For this review, take the finished solid that the model builds, in its own axes (mm). Face numbers are marked on the shaded views. A direction names the side the tool comes from. Coordinates: 2 decimals unless noted, no trailing zeros. Write each loop counter-clockwise with the first axis right and the second up, starting at its lowest first coordinate (ties: lowest second). Pieces come first, ordered by that corner, then holes.
1) We need section B-B on z = 32. Write out the cut boundary in (x, y), then the cut area to 3 significant figures.
2) We need section A-A on y = 0. Write out the cut boundary in (x, z), then the cut area to 3 significant figures.
3) We need section C-C on x = 73.5. Write out the cut boundary in (y, z).
4) We need section D-D on y = 67. Write out the cut boundary in (x, z).
5) Insertion check: P1, Ø8, axis at y = 56.5, z = 36.5, coming from the +X side; P2, Ø23.5, axis at x = 0, y = 0, coming from the -Z side; P3, Ø3, axis at x = -13, z = 6, coming from the -Y side; P4, Ø6, axis at x = -8.5, z = 33.5, coming from the -Y side. Each pin has a flat end and moves straight along its axis. Give the tip position at first contact, or say it passes through.
6) Mouldability with a two-part tool opening along Z and no side actions: class the marked faces 1, 2, 3 and 4 as pulls with the +Z half, pulls with the -Z half, needs draft (parallel to the pull), parting line crosses it, or undercut.
7) For the marked faces 5, 6, 7, 8 and 9, list the 3-axis set-ups (+Z, -Z, +X, -X, +Y, -Y) from which the entire face can be reached by the end or side of a thin tool; tool diameter is ignored.
8) To check wall thickness, follow line 1 along X through (y, z) = (-8, 46); line 2 along Y through (x, z) = (54, 7.5); line 3 along Z through (x, y) = (3, -2.5). State the ranges of each line that lie inside material, in increasing order.
from build123d import *

# Parameters (mm, degrees)
SKIZZE1_W                       = 50
SKIZZE1_H                       = 50
SKIZZE1_R                       = 45
AUFSATZ_LINEAR_AUSTRAGEN2_DEPTH = 55
SCHNITT_LINEAR_AUSTRAGEN1_DEPTH = 43
SKIZZE4_R                       = 1.5
SCHNITT_LINEAR_AUSTRAGEN2_DEPTH = 10
SKIZZE5_R                       = 3.5
SCHNITT_LINEAR_AUSTRAGEN3_DEPTH = 4.5
SCHNITT_LINEAR_AUSTRAGEN4_DEPTH = 21
SCHNITT_LINEAR_START            = -6
SKIZZE7_R                       = 13
SCHNITT_LINEAR_AUSTRAGEN5_DEPTH = 49
SKIZZE8_R                       = 12
SCHNITT_LINEAR_AUSTRAGEN6_DEPTH = 165.772570533
SKIZZE9_R                       = 1.65
SCHNITT_LINEAR_AUSTRAGEN9_DEPTH = 20


with BuildPart() as part:
    # Skizze1 → Aufsatz-Linear austragen2 (new body)
    with BuildSketch(Plane.XY):
        with BuildLine():
            Line((35, 35), (35, 85))
            Line((35, 85), (-27.896103401, 35.310160224))
            ThreePointArc((-27.896103401, 35.310160224), (19.617279971, 40.498917597), (45, 0))
            ThreePointArc((45, 0), (31.819805153, -31.819805153), (0, -45))
            Line((0, -45), (85, -45))
            Line((85, -45), (85, 35))
            Line((85, 35), (35, 35))
        make_face()
        with Locations((60, 60)):
            Rectangle(SKIZZE1_W, SKIZZE1_H)
        Circle(SKIZZE1_R)
    extrude(amount=AUFSATZ_LINEAR_AUSTRAGEN2_DEPTH)

    # Skizze3 → Schnitt-Linear austragen1 (cut)
    with BuildSketch(Plane.XZ.offset(45)):
        Polygon((60, 48.5), (19, 48.5), (19, 6.5), (60, 6.5), (60, 16.5), (70, 16.5), (70, 6.5), (85, 6.5), (85, 48.5), (70, 48.5), (70, 38.5), (60, 38.5), align=None)
    extrude(amount=-SCHNITT_LINEAR_AUSTRAGEN1_DEPTH, mode=Mode.SUBTRACT)

    # Skizze4 → Schnitt-Linear austragen2 (cut)
    with BuildSketch(Plane(origin=(70, 0, 0), x_dir=(0, 0, -1), z_dir=(1, 0, 0))):
        with Locations(Location((-42.999780644, -7.500219356, 0), (0, 0, 90))):
            Circle(SKIZZE4_R)
        with Locations(Location((-12.000219356, -7.500219356, 0), (0, 0, 90))):
            Circle(SKIZZE4_R)
        with Locations(Location((-12.000219356, -38.499780644, 0), (0, 0, 90))):
            Circle(SKIZZE4_R)
        with BuildLine():
            ThreePointArc((-41.499780644, -38.499780644), (-42.402127924, -37.123985882), (-44.023528946, -37.403450669))
            ThreePointArc((-44.023528946, -37.403450669), (-42.999780644, -38.499780644), (-41.903450669, -39.523528946))
            ThreePointArc((-41.903450669, -39.523528946), (-41.604342547, -39.050010158), (-41.499780644, -38.499780644))
        make_face()
        with BuildLine():
            ThreePointArc((-41.903450669, -39.523528946), (-42.999780644, -38.499780644), (-44.023528946, -37.403450669))
            ThreePointArc((-44.023528946, -37.403450669), (-44.060440815, -39.560440815), (-41.903450669, -39.523528946))
        make_face()
    extrude(amount=-SCHNITT_LINEAR_AUSTRAGEN2_DEPTH, mode=Mode.SUBTRACT)

    # Skizze5 → Schnitt-Linear austragen3 (cut)
    with BuildSketch(Plane(origin=(70, 0, 0), x_dir=(0, 0, -1), z_dir=(1, 0, 0))):
        with Locations(Location((-42.999780644, -7.500219356, 0), (0, 0, 90))):
            Circle(SKIZZE5_R)
        with Locations(Location((-12.000219356, -7.500219356, 0), (0, 0, 90))):
            Circle(SKIZZE5_R)
        with Locations(Location((-12.000219356, -38.499780644, 0), (0, 0, 90))):
            Circle(SKIZZE5_R)
        with Locations(Location((-42.999780644, -38.499780644, 0), (0, 0, 90))):
            Circle(SKIZZE5_R)
    extrude(amount=-SCHNITT_LINEAR_AUSTRAGEN3_DEPTH, mode=Mode.SUBTRACT)

    # Skizze6 → Schnitt-Linear austragen4 (cut, symmetric)
    with BuildSketch(Plane.XY.offset(27.5)):
        Polygon((29, 10.5), (19, 10.5), (19, 3), (19, -2), (29, -2), align=None)
        with BuildLine():
            Line((19, 3), (19, 10.5))
            Line((19, 10.5), (5.809475019, 10.5))
            ThreePointArc((5.809475019, 10.5), (9.486832981, 7.348469228), (11.618950039, 3))
            Line((11.618950039, 3), (19, 3))
        make_face()
    extrude(amount=SCHNITT_LINEAR_AUSTRAGEN4_DEPTH, both=True, mode=Mode.SUBTRACT)

    # Skizze7 → Schnitt-Linear austragen5 (cut)
    with BuildSketch(Plane.XY.offset(55).offset(SCHNITT_LINEAR_START)):
        Circle(SKIZZE7_R)
    extrude(amount=-SCHNITT_LINEAR_AUSTRAGEN5_DEPTH, mode=Mode.SUBTRACT)

    # Skizze8 → Schnitt-Linear austragen6 (cut, through all)
    with BuildSketch(Plane(origin=(85, 0, 0), x_dir=(0, 0, -1), z_dir=(1, 0, 0))):
        with Locations(Location((-27.5, 57.5, 0), (0, 0, 90))):
            Circle(SKIZZE8_R)
    extrude(amount=-SCHNITT_LINEAR_AUSTRAGEN6_DEPTH, mode=Mode.SUBTRACT)

    # Skizze9 → Schnitt-Linear austragen9 (cut)
    with BuildSketch(Plane(origin=(0, 0, 0), x_dir=(-1, 0, 0), z_dir=(0, 0, -1))):
        with Locations((-10.037587636, 14.335160775)):
            Circle(SKIZZE9_R)
        with Locations((14.335160775, 10.037587636)):
            Circle(SKIZZE9_R)
        with Locations((10.037587636, -14.335160775)):
            Circle(SKIZZE9_R)
        with Locations((-14.335160775, -10.037587636)):
            Circle(SKIZZE9_R)
    extrude(amount=-SCHNITT_LINEAR_AUSTRAGEN9_DEPTH, mode=Mode.SUBTRACT)


solid = part.part
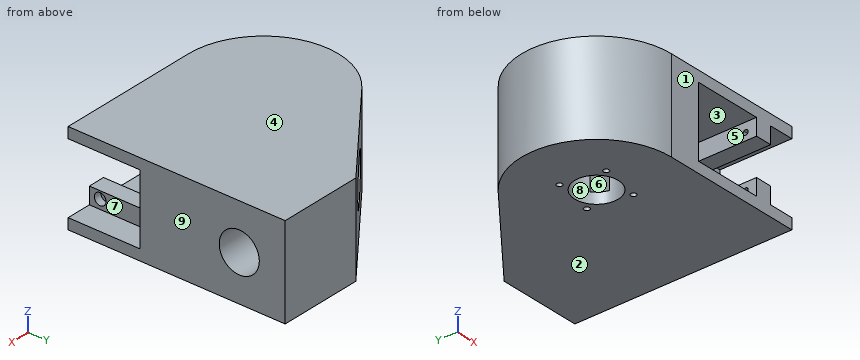
Result:
1. outline: (-27.9, 35.31) arc R45 ccw to (0, -45) - (19, -45) - (19, 3) - (12.65, 3) arc R13 cw (long way) to (7.66, 10.5) - (29, 10.5) - (29, -2) - (85, -2) - (85, 46.38) - (-13.89, 46.38) - close; (14.27, 68.62) - (85, 68.62) - (85, 85) - (35, 85) - close
1. area: 8,430 mm2
2. outline: (-45, 0) - (-13, 0) - (-13, 49) - (13, 49) - (13, 0) - (85, 0) - (85, 55) - (-45, 55) - close; hole (19, 6.5) - (29, 6.5) - (29, 48.5) - (19, 48.5) - close
2. area: 5,460 mm2
3. outline: (-45, 0) - (85, 0) - (85, 55) - (-45, 55) - (-45, 48.5) - (-2, 48.5) - (-2, 6.5) - (-45, 6.5) - close; hole circle Ø24 at (57.5, 27.5)
4. outline: (12.22, 0) - (85, 0) - (85, 20.17) - (12.22, 20.17) - close; (12.22, 34.83) - (85, 34.83) - (85, 55) - (12.22, 55) - close
5. P1: stops at x = 85
5. P2: stops at z = 49
5. P3: stops at y = -43.51
5. P4: stops at y = -44.66
6. face 1: needs draft
6. face 2: pulls with the -Z half
6. face 3: undercut
6. face 4: pulls with the +Z half
7. face 5: -Y
7. face 6: none
7. face 7: +X, -Y
7. face 8: -Z
7. face 9: +Z, -Z, +X, +Y, -Y
8. line 1: x = -44.28 to -10.25, 10.25 to 19, 60 to 65.5
8. line 2: y = -2 to 85
8. line 3: z = 49 to 55
